For this review, take the finished solid that the model builds, in its own axes (mm). Coordinates: 2 decimals unless noted, no trailing zeros. Loops run counter-clockwise (first coordinate to the right, second up) from the corner with the lowest first, then second, coordinate; pieces in that order, holes last. Notation, with made-up numbers: (81.25, 52) -> (112.25, 52) arc R25 cw to (112.25, 72) -> close; hole circle Ø2 at (41.25, -2.75). An arc over 180 degrees is marked (long way). Use a Markdown table: item, result.
from build123d import *

# Parameters (mm, degrees)
SKETCH_1_R      = 1.5
SKETCH_1_R_2    = 2
EXTRUDE_1_DEPTH = 5
FILLET_1_R      = 7
FILLET_4_R      = 5
FILLET_6_R      = 10


with BuildPart() as part:
    # 草图1 → 凸台-拉伸1 (new body)
    with BuildSketch(Plane(origin=(0, 0, 0), x_dir=(1, 0, 0), z_dir=(0, 1, 0))):
        with BuildLine():
            Line((0, 0), (160, 0))
            Line((160, 0), (160, -85))
            Line((160, -85), (170, -85))
            ThreePointArc((170, -85), (210, -125), (170, -165))
            Line((170, -165), (160, -165))
            Line((160, -165), (160, -250))
            Line((160, -250), (0, -250))
            Line((0, -250), (0, -159))
            Line((0, -159), (-50, -159))
            Line((-50, -159), (-50, -91))
            Line((-50, -91), (0, -91))
            Line((0, -91), (0, 0))
        make_face()
        with Locations(Location((154, -6, 0), (0, 0, 270))):
            Circle(SKETCH_1_R, mode=Mode.SUBTRACT)
        with Locations(Location((6, -6, 0), (0, 0, 90))):
            Circle(SKETCH_1_R, mode=Mode.SUBTRACT)
        with Locations(Location((152, -73, 0), (0, 0, 270))):
            Circle(SKETCH_1_R, mode=Mode.SUBTRACT)
        with Locations(Location((152, -177, 0), (0, 0, 90))):
            Circle(SKETCH_1_R, mode=Mode.SUBTRACT)
        with Locations(Location((154, -244, 0), (0, 0, 90))):
            Circle(SKETCH_1_R, mode=Mode.SUBTRACT)
        with Locations(Location((6, -244, 0), (0, 0, 270))):
            Circle(SKETCH_1_R, mode=Mode.SUBTRACT)
        with Locations(Location((50, -85, 0), (0, 0, 270))):
            Circle(SKETCH_1_R, mode=Mode.SUBTRACT)
        with Locations(Location((50, -165, 0), (0, 0, 90))):
            Circle(SKETCH_1_R, mode=Mode.SUBTRACT)
        with Locations(Location((13, -20, 0), (0, 0, 270))):
            Circle(SKETCH_1_R_2, mode=Mode.SUBTRACT)
        with Locations(Location((13, -200, 0), (0, 0, 270))):
            Circle(SKETCH_1_R_2, mode=Mode.SUBTRACT)
        with Locations(Location((20, -85, 0), (0, 0, 270))):
            Circle(SKETCH_1_R, mode=Mode.SUBTRACT)
        with Locations(Location((20, -165, 0), (0, 0, 90))):
            Circle(SKETCH_1_R, mode=Mode.SUBTRACT)
        with Locations(Location((89, -88, 0), (0, 0, 270))):
            Circle(SKETCH_1_R, mode=Mode.SUBTRACT)
        with Locations(Location((126, -88, 0), (0, 0, 270))):
            Circle(SKETCH_1_R, mode=Mode.SUBTRACT)
        with Locations(Location((126, -155, 0), (0, 0, 270))):
            Circle(SKETCH_1_R, mode=Mode.SUBTRACT)
        with Locations(Location((89, -155, 0), (0, 0, 270))):
            Circle(SKETCH_1_R, mode=Mode.SUBTRACT)
        with Locations(Location((43, -200, 0), (0, 0, 270))):
            Circle(SKETCH_1_R_2, mode=Mode.SUBTRACT)
        with Locations(Location((13, -230, 0), (0, 0, 270))):
            Circle(SKETCH_1_R_2, mode=Mode.SUBTRACT)
        with Locations(Location((43, -230, 0), (0, 0, 270))):
            Circle(SKETCH_1_R_2, mode=Mode.SUBTRACT)
        with Locations(Location((117, -230, 0), (0, 0, 90))):
            Circle(SKETCH_1_R_2, mode=Mode.SUBTRACT)
        with Locations(Location((147, -230, 0), (0, 0, 90))):
            Circle(SKETCH_1_R_2, mode=Mode.SUBTRACT)
        with Locations(Location((117, -200, 0), (0, 0, 90))):
            Circle(SKETCH_1_R_2, mode=Mode.SUBTRACT)
        with Locations(Location((147, -200, 0), (0, 0, 90))):
            Circle(SKETCH_1_R_2, mode=Mode.SUBTRACT)
        with Locations(Location((43, -20, 0), (0, 0, 270))):
            Circle(SKETCH_1_R_2, mode=Mode.SUBTRACT)
        with Locations(Location((13, -50, 0), (0, 0, 270))):
            Circle(SKETCH_1_R_2, mode=Mode.SUBTRACT)
        with Locations(Location((43, -50, 0), (0, 0, 270))):
            Circle(SKETCH_1_R_2, mode=Mode.SUBTRACT)
        with Locations(Location((117, -20, 0), (0, 0, 90))):
            Circle(SKETCH_1_R_2, mode=Mode.SUBTRACT)
        with Locations(Location((117, -50, 0), (0, 0, 90))):
            Circle(SKETCH_1_R_2, mode=Mode.SUBTRACT)
        with Locations(Location((147, -50, 0), (0, 0, 90))):
            Circle(SKETCH_1_R_2, mode=Mode.SUBTRACT)
        with Locations(Location((147, -20, 0), (0, 0, 90))):
            Circle(SKETCH_1_R_2, mode=Mode.SUBTRACT)
        with Locations(Location((145.605, -100.605, 0), (0, 0, 270))):
            Circle(SKETCH_1_R, mode=Mode.SUBTRACT)
        with Locations(Location((194.395, -100.605, 0), (0, 0, 270))):
            Circle(SKETCH_1_R, mode=Mode.SUBTRACT)
        with Locations(Location((194.395, -149.395, 0), (0, 0, 270))):
            Circle(SKETCH_1_R, mode=Mode.SUBTRACT)
        with Locations(Location((145.605, -149.395, 0), (0, 0, 270))):
            Circle(SKETCH_1_R, mode=Mode.SUBTRACT)
    extrude(amount=EXTRUDE_1_DEPTH)

    # 圆角1
    fillet_1_edges = [part.edges().sort_by_distance(p)[0] for p in [
        (0, 2.5, 0),
        (160, 2.5, 0),
        (160, 2.5, 250),
        (0, 2.5, 250),
        (-50, 2.5, 159),
        (-50, 2.5, 91),
    ]]
    fillet(fillet_1_edges, radius=FILLET_1_R)

    # 圆角4
    fillet_4_edges = [part.edges().sort_by_distance(p)[0] for p in [
        (0, 2.5, 159),
        (0, 2.5, 91),
    ]]
    fillet(fillet_4_edges, radius=FILLET_4_R)

    # 圆角6
    fillet_6_edges = [part.edges().sort_by_distance(p)[0] for p in [
        (160, 2.5, 85),
        (160, 2.5, 165),
    ]]
    fillet(fillet_6_edges, radius=FILLET_6_R - 0.0001)  # a hair under: the kernel refuses the full size


solid = part.part
(1) For line 1 along Z through (x, y) = (152, 1.6); line 2 along Z through (x, y) = (117, 2.2); line 3 along X through (y, z) = (1.9, 200), list the stretches that pass through material, from the lowest coordinate up.
Found:
| item | result |
|---|---|
| line 1 | z = 0 to 71.5, 74.5 to 175.5, 178.5 to 250 |
| line 2 | z = 0 to 18, 22 to 48, 52 to 198, 202 to 228, 232 to 250 |
| line 3 | x = 0 to 11, 15 to 41, 45 to 115, 119 to 145, 149 to 160 |
(2) Take a section at B-B on z = 33. Write out the cut boundary in (x, y).
Found:
| item | result |
|---|---|
| outline | (0, 0) -> (160, 0) -> (160, 5) -> (0, 5) -> close |
(3) For pin 1 Ø1.5 at (y, z) = (3.5, 54.5) entering from -X; pin 2 Ø1.5 at (x, y) = (-21.5, 2) entering from -Z, all flat-tipped, find the tip position at first contact; note any pin that passes through.
Found:
| item | result |
|---|---|
| pin 1 | stops at x = 0 |
| pin 2 | stops at z = 91 |
(4) Take a section at A-A on x = -25. Write out the cut boundary in (y, z), plus the area to 3 significant figures.
Found:
| item | result |
|---|---|
| outline | (0, 91) -> (5, 91) -> (5, 159) -> (0, 159) -> close |
| area | 340 mm^2 |
